For this review, take the finished solid that the model builds, in its own axes (mm). Face numbers are marked on the shaded views. A direction names the side the tool comes from. Coordinates: 2 decimals unless noted, no trailing zeros. Loops run counter-clockwise (first coordinate to the right, second up) from the corner with the lowest first, then second, coordinate; pieces in that order, holes last. Notation, with made-up numbers: (19.5, 29.25) -> (49.5, 29.25) arc R17 ccw to (49.5, 55.25) -> close; hole circle Ø7 at (-11, 73.25). An arc over 180 degrees is marked (long way). Use a Markdown table: item, result.
from build123d import *

# Parameters (mm, degrees)
F0_W         = 30
F0_H         = 35
F1_DEPTH     = 13
F2_W         = 3.9074438825
F2_H         = 9.5
F3_DEPTH     = 35.001
F4_W         = 2.524356873
F4_H         = 7
F5_DEPTH     = 35.001
F6_R         = 5
F8_DEPTH     = 30.001
F9_R         = 1.5246036127
F10_DEPTH    = 10.501
F11_T1_DEPTH = 42.5
F11_T3_DEPTH = 38.085325067


# Not quite as in the source:
# - a fillet or chamfer that OpenCascade refuses, or shapes differently, is made with other operations: its cross-section is extruded or revolved along the edge and cut away or added


with BuildPart() as f1:
    # F0 (on Top) → F1 (new body)
    with BuildSketch(Plane.XY):
        with Locations((15, 17.5)):
            Rectangle(F0_W, F0_H)
    extrude(amount=F1_DEPTH)

    # F2 (on face) → F3 (cut, through all)
    with BuildSketch(Plane.XZ):
        with Locations((1.9537219413, 8.25)):
            Rectangle(F2_W, F2_H)
        Polygon((15, 13), (5.4074438825, 13), (15, 3.5), (24.5925561175, 13), align=None)
        with Locations((28.0462780587, 8.25)):
            Rectangle(F2_W, F2_H)
    extrude(amount=-F3_DEPTH, mode=Mode.SUBTRACT)

    # F4 (on face) → F5 (cut, through all)
    with BuildSketch(Plane.XZ):
        Polygon((6.4318007555, 10.5), (7.9318007555, 10.5), (5.4074438825, 13), (3.9074438825, 13), (3.9074438825, 10.5), align=None)
        Polygon((23.5681992445, 10.5), (26.0925561175, 10.5), (26.0925561175, 13), (24.5925561175, 13), (22.0681992445, 10.5), align=None)
        with Locations((5.169622319, 7)):
            Rectangle(F4_W, F4_H)
        with Locations((24.830377681, 7)):
            Rectangle(F4_W, F4_H)
    extrude(amount=-F5_DEPTH, mode=Mode.SUBTRACT)

    # F6
    f6_edges = [f1.edges().sort_by_distance(p)[0] for p in [
        (15, 17.5, 3.5),
    ]]
    fillet(f6_edges, radius=F6_R)

    # F7 (on face) → F8 (cut, through all)
    with BuildSketch(Plane(origin=(0, 0, 0), x_dir=(0, -1, 0), z_dir=(-1, 0, 0))):
        with BuildLine():
            ThreePointArc((-15, 3.5), (-17.5, 6), (-20, 3.5))
            Line((-20, 3.5), (-15, 3.5))
        make_face()
    extrude(amount=-F8_DEPTH, mode=Mode.SUBTRACT)

    # F9 (on face) → F10 (cut, through all)
    with BuildSketch(Plane(origin=(0, 0, 0), x_dir=(1, 0, 0), z_dir=(0, 0, -1))):
        with Locations((3.3, -3.75)):
            Circle(F9_R)
        with Locations((26.7, -3.75)):
            Circle(F9_R)
        with Locations((3.3, -31.25)):
            Circle(F9_R)
        with Locations((26.7, -31.25)):
            Circle(F9_R)
    extrude(amount=-F10_DEPTH, mode=Mode.SUBTRACT)

    # F11: fillet of radius 1.5 on 3 edges, made by hand

    # F11_s2 → F11_t1 (cut)
    with BuildSketch(Plane.XZ.offset(-38.75)):
        with BuildLine():
            ThreePointArc((7.9318007555, 10.5), (6.8711405838, 10.0606601718), (6.4318007555, 9))
            Line((6.4318007555, 9), (6.4318007555, 10.5))
            Line((6.4318007555, 10.5), (7.9318007555, 10.5))
        make_face()
        with BuildLine():
            ThreePointArc((22.0681992445, 10.5), (23.1288594162, 10.0606601718), (23.5681992445, 9))
            Line((23.5681992445, 9), (23.5681992445, 10.5))
            Line((23.5681992445, 10.5), (22.0681992445, 10.5))
        make_face()
    extrude(amount=F11_T1_DEPTH, mode=Mode.SUBTRACT)

    # F11_s4 → F11_t3 (cut)
    with BuildSketch(Plane.XZ.offset(-36.5426625335)):
        with BuildLine():
            ThreePointArc((21.6297583139, 10.0657894737), (22.1145998252, 10.3872065835), (22.6852642579, 10.5))
            Line((22.6852642579, 10.5), (22.0681992445, 10.5))
            Line((22.0681992445, 10.5), (21.6297583139, 10.0657894737))
        make_face()
    extrude(amount=F11_T3_DEPTH, mode=Mode.SUBTRACT)


solid = f1.part
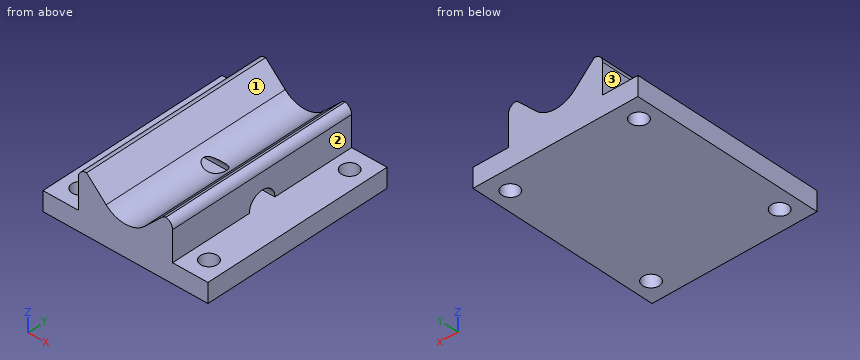
(1) For line 1 along X through (y, z) = (3.75, 0.95); line 2 along Y through (x, z) = (3.3, 1.2); line 3 along Z through (x, y) = (28.5, 2), list the stretches that pass through material, from the lowest coordinate up.
Found:
| item | result |
|---|---|
| line 1 | x = 0 to 1.78, 4.82 to 25.18, 28.22 to 30 |
| line 2 | y = 0 to 2.23, 5.27 to 29.73, 32.77 to 35 |
| line 3 | z = 0 to 3.5 |
(2) Take a section at A-A on x = 26.7. Write out the cut boundary in (y, z), plus the area to 3 significant figures.
Found:
| item | result |
|---|---|
| outline | (0, 0) -> (2.23, 0) -> (2.23, 3.5) -> (0, 3.5) -> close; (5.27, 0) -> (29.73, 0) -> (29.73, 3.5) -> (5.27, 3.5) -> close; (32.77, 0) -> (35, 0) -> (35, 3.5) -> (32.77, 3.5) -> close |
| area | 101 mm^2 |
(3) Take a section at B-B on y = 3.75. Write out the cut boundary in (x, z).
Found:
| item | result |
|---|---|
| outline | (0, 0) -> (1.78, 0) -> (1.78, 3.5) -> (0, 3.5) -> close; (4.82, 0) -> (25.18, 0) -> (25.18, 3.5) -> (23.57, 3.5) -> (23.57, 9) arc R1.5 ccw to (22.38, 10.47) arc R1.5 ccw to (21.63, 10.07) -> (18.52, 6.98) arc R5 cw to (11.48, 6.98) -> (7.93, 10.5) arc R1.5 ccw to (6.43, 9) -> (6.43, 3.5) -> (4.82, 3.5) -> close; (28.22, 0) -> (30, 0) -> (30, 3.5) -> (28.22, 3.5) -> close |
(4) Take a section at D-D on z = 9.5. Write out the cut boundary in (x, y).
Found:
| item | result |
|---|---|
| outline | (6.52, 0) -> (8.94, 0) -> (8.94, 35) -> (6.52, 35) -> close; (21.06, 0) -> (23.48, 0) -> (23.48, 35) -> (21.06, 35) -> close |
(5) For the marked faces 1, 2 and 3, list the 3-axis set-ups (+Z, -Z, +X, -X, +Y, -Y) from which the entire face can be reached by the end or side of a thin tool; tool diameter is ignored.
Found:
| item | result |
|---|---|
| face 1 | +Z, +Y, -Y |
| face 2 | +Z, +X, +Y, -Y |
| face 3 | +Z, -X, +Y, -Y |
(6) Take a section at C-C on z = 3. Write out the cut boundary in (x, y), plus the area to 3 significant figures.
Found:
| item | result |
|---|---|
| outline | (0, 0) -> (30, 0) -> (30, 35) -> (0, 35) -> close; hole circle Ø3.05 at (3.3, 3.75); hole circle Ø3.05 at (3.3, 31.25); hole circle Ø3.05 at (26.7, 3.75); hole circle Ø3.05 at (26.7, 31.25) |
| area | 1,020 mm^2 |
(7) For pin 1 Ø1.6 at (y, z) = (15, 6.5) entering from +X; pin 2 Ø9 at (x, y) = (12.5, 19.5) entering from +Z; pin 3 Ø5 at (x, y) = (26.7, 3.75) entering from +Z, all flat-tipped, find the tip position at first contact; note any pin that passes through.
Found:
| item | result |
|---|---|
| pin 1 | stops at x = 23.57 |
| pin 2 | stops at z = 10.43 |
| pin 3 | stops at z = 3.5 |
